Can you work these out from the model? Positions are in its coordinate system, mm. Face numbers are marked on the shaded views. A direction names the side the tool comes from. Give positions to 0.01 mm unless a question says otherwise; leave off trailing zeros. Write each loop counter-clockwise with the first axis right and the second up, starting at its lowest first coordinate (ties: lowest second). Pieces come first, ordered by that corner, then holes.
1. On a 3-axis mill with a long thin cutter (end or side, diameter ignored), from which of +Z, -Z, +X, -X, +Y, -Y can I reach the whole of each face in a straight line? I mean the marked faces 4 and 5. Say none if no direction works.
2. Suppose I cut it at C-C (x = 20). Please give me the cut outline in (y, z), and give its area (3 significant figures).
3. I'm going to push flat-ended pins straight in: pin 1 (5 mm diameter, centred on x = 9.5, y = 17, fed in from -Z); pin 2 (5 mm diameter, centred on x = 6, z = 7.5, fed in from +Y); pin 3 (1.8 mm diameter, centred on x = 2.795, y = 25, fed in from -Z); pin 4 (5 mm diameter, centred on x = 10, y = 25, fed in from +Z). Where does each tip first touch, or does it pass through?
4. Suppose I cut it at A-A (x = 10). Please give me the cut outline in (y, z), and give its area (3 significant figures).
5. Suppose I cut it at B-B (z = 19). Please give me the cut outline in (x, y), and give its area (3 significant figures).
6. Suppose I cut it at D-D (y = 11.5). Please give me the cut outline in (x, z).
7. If I drill on probe 1 along Z at (x, y) = (-20, -1); probe 2 along Y at (x, z) = (10, -25.1); probe 3 along Z at (x, y) = (1, 8), over which ranges is the centre line in solid material (lowest first)?
8. Thinking about a two-plate mould opening in Z: for the marked faces 1, 2 and 3, which applies, pulls with the +Z half, pulls with the -Z half, needs draft (parallel to the pull), parting line crosses it, or undercut?
```python
from build123d import *

# Parameters (mm, degrees)
SKETCH_W     = 50
SKETCH_H     = 48
SKETCH_R     = 1.5
PAD_DEPTH    = 2
SKETCH003_R  = 1.5
PAD001_DEPTH = 2
SKETCH004_R  = 3.5
PAD002_DEPTH = 2
FILLET_R     = 1
FILLET001_R  = 1


with BuildPart() as part:
    # Sketch → Pad (new body)
    with BuildSketch(Plane.XZ):
        Rectangle(SKETCH_W, SKETCH_H)
        with Locations((-20, 19)):
            Circle(SKETCH_R, mode=Mode.SUBTRACT)
        with Locations((20, 19)):
            Circle(SKETCH_R, mode=Mode.SUBTRACT)
        with Locations((-20, -19)):
            Circle(SKETCH_R, mode=Mode.SUBTRACT)
        with Locations((20, -19)):
            Circle(SKETCH_R, mode=Mode.SUBTRACT)
    extrude(amount=PAD_DEPTH)

    # Sketch003 (on Face3 of Pad) → Pad001 (join)
    with BuildSketch(Plane(origin=(0, 0, -24), x_dir=(1, 0, 0), z_dir=(0, 0, -1))):
        with BuildLine():
            Line((-25, 0), (-25, 2))
            Line((-25, 2), (25, 2))
            Line((25, 2), (25, 0))
            Line((25, 0), (25, -5))
            Line((25, -5), (20.80638, -27.054785))
            ThreePointArc((1.756653, -32.283353), (12.911489, -35.607697), (20.80638, -27.054785))
            Line((-25, -2), (1.756653, -32.283353))
            Line((-25, 0), (-25, -2))
        make_face()
        with Locations((10, -31.934549)):
            Circle(SKETCH003_R, mode=Mode.SUBTRACT)
        with Locations((17.205, -25)):
            Circle(SKETCH003_R, mode=Mode.SUBTRACT)
        with Locations((10, -25)):
            Circle(SKETCH003_R, mode=Mode.SUBTRACT)
        with Locations((2.795, -25)):
            Circle(SKETCH003_R, mode=Mode.SUBTRACT)
        with Locations((10, -18.065451)):
            Circle(SKETCH003_R, mode=Mode.SUBTRACT)
    extrude(amount=PAD001_DEPTH)

    # Sketch004 (on Face1 of Pad) → Pad002 (join)
    with BuildSketch(Plane(origin=(0, 0, 24), x_dir=(-1, 0, 0), z_dir=(0, 0, 1))):
        with BuildLine():
            Line((-25, 2), (25, 2))
            Line((25, 2), (25, 0))
            Line((25, 0), (25, -2))
            Line((25, -2), (-1.756653, -32.283353))
            ThreePointArc((-20.80638, -27.054785), (-12.911489, -35.607697), (-1.756653, -32.283353))
            Line((-25, -5), (-20.80638, -27.054785))
            Line((-25, 0), (-25, -5))
            Line((-25, 0), (-25, 2))
        make_face()
        with Locations((-10, -25)):
            Circle(SKETCH004_R, mode=Mode.SUBTRACT)
    extrude(amount=PAD002_DEPTH)

    # Fillet
    fillet_edges = [part.edges().sort_by_distance(p)[0] for p in [
        (0, 0, -24),
    ]]
    fillet(fillet_edges, radius=FILLET_R)

    # Fillet001
    fillet001_edges = [part.edges().sort_by_distance(p)[0] for p in [
        (0, 0, 24),
    ]]
    fillet(fillet001_edges, radius=FILLET001_R)


solid = part.part
```
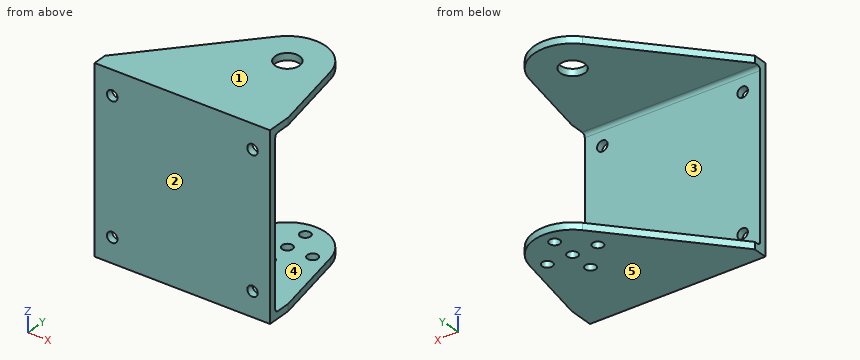
Checks:
1. face 4: +X, -X, +Y
1. face 5: -Z, +X, -X, +Y, -Y
2. outline: (-2, -26) - (29.58, -26) - (29.58, -24) - (1, -24) arc R1 cw to (0, -23) - (0, -20.5) - (-2, -20.5) - close; (-2, -17.5) - (0, -17.5) - (0, 17.5) - (-2, 17.5) - close; (-2, 20.5) - (0, 20.5) - (0, 23) arc R1 cw to (1, 24) - (29.58, 24) - (29.58, 26) - (-2, 26) - close
2. area: 211 mm2
3. pin 1: stops at z = -26
3. pin 2: stops at y = 0
3. pin 3: stops at z = 24
3. pin 4: stops at z = -24
4. outline: (-2, -26) - (16.57, -26) - (16.57, -24) - (1, -24) arc R1 cw to (0, -23) - (0, 23) arc R1 cw to (1, 24) - (21.5, 24) - (21.5, 26) - (-2, 26) - close; (19.57, -26) - (23.5, -26) - (23.5, -24) - (19.57, -24) - close; (26.5, -26) - (30.43, -26) - (30.43, -24) - (26.5, -24) - close; (28.5, 24) - (36, 24) - (36, 26) - (28.5, 26) - close; (33.43, -26) - (36, -26) - (36, -24) - (33.43, -24) - close
4. area: 216 mm2
5. outline: (-25, -2) - (-21.5, -2) - (-21.5, 0) - (-25, 0) - close; (-18.5, -2) - (18.5, -2) - (18.5, 0) - (-18.5, 0) - close; (21.5, -2) - (25, -2) - (25, 0) - (21.5, 0) - close
5. area: 88.0 mm2
6. outline: (-16.61, -26) - (23.76, -26) - (23.76, -24) - (-16.61, -24) - close; (-16.61, 24) - (23.76, 24) - (23.76, 26) - (-16.61, 26) - close
7. probe 1: z = -26 to -20.5, -17.5 to 17.5, 20.5 to 26
7. probe 2: y = -2 to 16.57, 19.57 to 23.5, 26.5 to 30.43, 33.43 to 36
7. probe 3: z = -26 to -24, 24 to 26
8. face 1: pulls with the +Z half
8. face 2: needs draft
8. face 3: undercut
